The listing builds one solid part. Answer for the finished solid, in the listing's coordinates (mm). A direction names the side the tool comes from. Round coordinates to 2 decimals unless told otherwise and drop trailing zeros. Write each loop counter-clockwise with the first axis right and the second up, starting at its lowest first coordinate (ties: lowest second). Pieces come first, ordered by that corner, then holes.
Item 1: Each of these flat-tipped pins is pushed along its axis until it touches: pin 1 (5 mm diameter, centred on x = 10, z = 3.5, fed in from -Y); pin 2 (2 mm diameter, centred on y = 1, z = -15, fed in from -X); pin 3 (5 mm diameter, centred on y = 9, z = -2, fed in from +X); pin 4 (1 mm diameter, centred on x = -1.5, z = 10, fed in from +Y). Where does it stop, or does it pass through?
Item 2: Find section B-B on x = 1.75. Give the vertices of the cut face in (y, z).
Item 3: For a pull along Z with two mould halves and no side action, classify faces 4 (the face through (6.817, 6.902, -3.945)), 5 (the face through (0, 10.5, 6.7)), 6 (the face through (7.88, 5.797, -18.409)) as +Z half, -Z half, draft (parallel to the pull), parting line (faces both ways), or undercut.
Item 4: Find section A-A on x = 8. Give the vertices of the cut face in (y, z), then the cut area to 3 significant figures.
Item 5: Find the intervals of material crossed by probe 1 along X at (y, z) = (-2.5, 7.5); probe 2 along Y at (x, z) = (0.65, 0); probe 3 along Y at (x, z) = (6.25, 0), in increasing order.
Item 6: A tool of negligible diameter and unlimited length cuts with its end or side. For faces 1 (the face through (12.8, -2.1, -4.4)), 2 (the face through (6.817, 4.513, 4.27)), 3 (the face through (0.5, -12, -2.7)), from which of +Z, -Z, +X, -X, +Y, -Y can it reach the whole face along a straight path? Write none if from no direction.
```python
from build123d import *

# Parameters (mm, degrees)
ESQUISSE1_R             = 19.3
EXTRUSION1_DEPTH        = 15.8
ESQUISSE2_R             = 12.3
ENL_V_MAT_EXTRU_1_DEPTH = 1
ESQUISSE3_R             = 11.3
ENL_V_MAT_EXTRU_2_DEPTH = 1
ESQUISSE4_R             = 10.3
ENL_V_MAT_EXTRU_3_DEPTH = 1
ESQUISSE6_R             = 12.3
ENL_V_MAT_EXTRU_4_DEPTH = 1
ESQUISSE7_R             = 4.5
EXTRUSION3_DEPTH        = 5
ESQUISSE8_R             = 4.5
EXTRUSION4_DEPTH        = 1
ESQUISSE9_R             = 1.5
ENL_V_MAT_EXTRU_5_DEPTH = 18.8
CONG_1_R                = 6.5


with BuildPart() as part:
    # Esquisse1 → Extrusion1 (new body)
    with BuildSketch(Plane(origin=(0, 0, 0), x_dir=(0, 0, -1), z_dir=(1, 0, 0))):
        Circle(ESQUISSE1_R)
        with BuildLine():
            Line((1.9, 4.079215611), (1.65, 7.776888838))
            ThreePointArc((1.65, 7.776888838), (3.975, 6.88490196), (5.909983296, 5.317386335))
            Line((5.909983296, 5.317386335), (2.582704347, 3.685056073))
            ThreePointArc((2.582704347, 3.685056073), (2.25, 3.897114317), (1.9, 4.079215611))
        make_face(mode=Mode.SUBTRACT)
        with BuildLine():
            Line((-1.9, 4.079215611), (-1.65, 7.776888838))
            ThreePointArc((-1.65, 7.776888838), (-3.975, 6.88490196), (-5.909983296, 5.317386335))
            Line((-5.909983296, 5.317386335), (-2.582704347, 3.685056073))
            ThreePointArc((-2.582704347, 3.685056073), (-2.25, 3.897114317), (-1.9, 4.079215611))
        make_face(mode=Mode.SUBTRACT)
        with BuildLine():
            Line((4.482704347, 0.394159538), (7.559983296, 2.459502503))
            ThreePointArc((7.559983296, 2.459502503), (7.95, 0), (7.559983296, -2.459502503))
            Line((7.559983296, -2.459502503), (4.482704347, -0.394159538))
            ThreePointArc((4.482704347, -0.394159538), (4.5, 0), (4.482704347, 0.394159538))
        make_face(mode=Mode.SUBTRACT)
        with BuildLine():
            Line((2.582704347, -3.685056073), (5.909983296, -5.317386335))
            ThreePointArc((5.909983296, -5.317386335), (3.975, -6.88490196), (1.65, -7.776888838))
            Line((1.65, -7.776888838), (1.9, -4.079215611))
            ThreePointArc((1.9, -4.079215611), (2.25, -3.897114317), (2.582704347, -3.685056073))
        make_face(mode=Mode.SUBTRACT)
        with BuildLine():
            Line((-1.9, -4.079215611), (-1.65, -7.776888838))
            ThreePointArc((-1.65, -7.776888838), (-3.975, -6.88490196), (-5.909983296, -5.317386335))
            Line((-5.909983296, -5.317386335), (-2.582704347, -3.685056073))
            ThreePointArc((-2.582704347, -3.685056073), (-2.25, -3.897114317), (-1.9, -4.079215611))
        make_face(mode=Mode.SUBTRACT)
        with BuildLine():
            Line((-4.482704347, -0.394159538), (-7.559983296, -2.459502503))
            ThreePointArc((-7.559983296, -2.459502503), (-7.95, 0), (-7.559983296, 2.459502503))
            Line((-7.559983296, 2.459502503), (-4.482704347, 0.394159538))
            ThreePointArc((-4.482704347, 0.394159538), (-4.5, 0), (-4.482704347, -0.394159538))
        make_face(mode=Mode.SUBTRACT)
    extrude(amount=EXTRUSION1_DEPTH)

    # Esquisse2 → Enlèv. mat.-Extru.1 (cut)
    with BuildSketch(Plane(origin=(15.8, 0, 0), x_dir=(0, 0, -1), z_dir=(1, 0, 0))):
        Circle(ESQUISSE2_R)
    extrude(amount=-ENL_V_MAT_EXTRU_1_DEPTH, mode=Mode.SUBTRACT)

    # Esquisse3 → Enlèv. mat.-Extru.2 (cut)
    with BuildSketch(Plane(origin=(14.8, 0, 0), x_dir=(0, 0, -1), z_dir=(1, 0, 0))):
        Circle(ESQUISSE3_R)
    extrude(amount=-ENL_V_MAT_EXTRU_2_DEPTH, mode=Mode.SUBTRACT)

    # Esquisse4 → Enlèv. mat.-Extru.3 (cut)
    with BuildSketch(Plane(origin=(13.8, 0, 0), x_dir=(0, 0, -1), z_dir=(1, 0, 0))):
        Circle(ESQUISSE4_R)
    extrude(amount=-ENL_V_MAT_EXTRU_3_DEPTH, mode=Mode.SUBTRACT)

    # Esquisse6 → Enlèv. mat.-Extru.4 (cut)
    with BuildSketch(Plane.ZY):
        Circle(ESQUISSE6_R)
    extrude(amount=-ENL_V_MAT_EXTRU_4_DEPTH, mode=Mode.SUBTRACT)

    # Esquisse7 → Extrusion3 (add)
    with BuildSketch(Plane.ZY.offset(-1)):
        Circle(ESQUISSE7_R)
    extrude(amount=EXTRUSION3_DEPTH)

    # Esquisse8 → Extrusion4 (add)
    with BuildSketch(Plane(origin=(12.8, 0, 0), x_dir=(0, 0, -1), z_dir=(1, 0, 0))):
        Circle(ESQUISSE8_R)
    extrude(amount=EXTRUSION4_DEPTH)

    # Esquisse9 → Enlèv. mat.-Extru.5 (cut, through all)
    with BuildSketch(Plane(origin=(13.8, 0, 0), x_dir=(0, 0, -1), z_dir=(1, 0, 0))):
        Circle(ESQUISSE9_R)
    extrude(amount=-ENL_V_MAT_EXTRU_5_DEPTH, mode=Mode.SUBTRACT)

    # Congé1
    cong_1_edges = [part.edges().sort_by_distance(p)[0] for p in [
        (0, 0, 19.3),
        (15.8, 0, 19.3),
    ]]
    fillet(cong_1_edges, radius=CONG_1_R)


solid = part.part
```
Check values:
1. pin 1: stops at y = -19.27
1. pin 2: stops at x = 0.12
1. pin 3: stops at x = 14.8
1. pin 4: passes through
2. outline: circle Ø34.47 at (0, 0); hole (-7.78, -1.65) arc R7.95 ccw to (-5.32, -5.91) - (-3.69, -2.58) arc R4.5 cw to (-4.08, -1.9) - close; hole (-7.78, 1.65) - (-4.08, 1.9) arc R4.5 cw to (-3.69, 2.58) - (-5.32, 5.91) arc R7.95 ccw to start; hole (-2.46, -7.56) arc R7.95 ccw to (2.46, -7.56) - (0.39, -4.48) arc R4.5 cw to (-0.39, -4.48) - close; hole (-2.46, 7.56) - (-0.39, 4.48) arc R4.5 cw to (0.39, 4.48) - (2.46, 7.56) arc R7.95 ccw to start; hole circle Ø3 at (0, 0); hole (3.69, -2.58) - (5.32, -5.91) arc R7.95 ccw to (7.78, -1.65) - (4.08, -1.9) arc R4.5 cw to start; hole (3.69, 2.58) arc R4.5 cw to (4.08, 1.9) - (7.78, 1.65) arc R7.95 ccw to (5.32, 5.91) - close
3. face 4: undercut
3. face 5: draft
3. face 6: parting line
4. outline: circle Ø38.6 at (0, 0); hole (-7.78, -1.65) arc R7.95 ccw to (-5.32, -5.91) - (-3.69, -2.58) arc R4.5 cw to (-4.08, -1.9) - close; hole (-7.78, 1.65) - (-4.08, 1.9) arc R4.5 cw to (-3.69, 2.58) - (-5.32, 5.91) arc R7.95 ccw to start; hole (-2.46, -7.56) arc R7.95 ccw to (2.46, -7.56) - (0.39, -4.48) arc R4.5 cw to (-0.39, -4.48) - close; hole (-2.46, 7.56) - (-0.39, 4.48) arc R4.5 cw to (0.39, 4.48) - (2.46, 7.56) arc R7.95 ccw to start; hole circle Ø3 at (0, 0); hole (3.69, -2.58) - (5.32, -5.91) arc R7.95 ccw to (7.78, -1.65) - (4.08, -1.9) arc R4.5 cw to start; hole (3.69, 2.58) arc R4.5 cw to (4.08, 1.9) - (7.78, 1.65) arc R7.95 ccw to (5.32, 5.91) - close
4. area: 1,100 mm2
5. probe 1: x = 1 to 12.8
5. probe 2: y = -15.63 to -12.3, -4.5 to -1.5, 1.5 to 4.5, 12.3 to 15.63
5. probe 3: y = -19.3 to -1.5, 1.5 to 19.3
6. face 1: +X
6. face 2: +X, -X
6. face 3: -X
